Check sheet for the modelled part. Datum: model origin and axes. Units: mm. Coordinates: 2 decimals unless noted, no trailing zeros. Order: outer loops, then holes, each group sorted by start corner. A loop starts at its lowest first (then second) coordinate and runs counter-clockwise, first axis right, second up. Notation, with made-up numbers: (55, 48) -> (109, 48) arc R31 cw to (109, 82) -> close; hole circle Ø10 at (-6, 82). An arc over 180 degrees is marked (long way). Put each result on its own line as item: value. Start each with the question number.
```python
from build123d import *

# Parameters (mm, degrees)
F1_DEPTH = 6.35
F3_D     = 4.4958


with BuildPart() as f1:
    # F0 (on Front) → F1 (new body)
    with BuildSketch(Plane.XZ):
        with BuildLine():
            Line((18.2969275085, 15.24), (-18.2969275085, 15.24))
            ThreePointArc((-18.2969275085, 15.24), (0, -23.8125), (18.2969275085, 15.24))
        make_face()
    extrude(amount=F1_DEPTH)

    # F3 (through all)
    with Locations(Plane.XZ.offset(6.35)):
        with Locations((-15.7602855304, 9.525), (15.7602855304, 9.525), (-9.525, -15.7602855304), (9.525, -15.7602855304)):
            Hole(F3_D / 2)


solid = f1.part
```
1) Scan lines: line 1 along X through (y, z) = (-3.25, 8.5); line 2 along X through (y, z) = (-3.5, 9); line 3 along Z through (x, y) = (-17.5, -3). Record each from-to range of solid material in increasing order. Write a range as [from, to].
2) Sectioned sample at B-B (z = 8). Record the boundary of the cut face in (x, y).
3) Gauge pin test, flat ends, axial feed: pin 1 (1.5 mm diameter, centred on y = -2.5, z = 5, fed in from -X); pin 2 (3.5 mm diameter, centred on x = 15.76, z = 9.52, fed in from +Y); pin 3 (3 mm diameter, centred on y = -5.5, z = 7, fed in from +X); pin 4 (1 mm diameter, centred on y = -4, z = 1.5, fed in from +X). Record the tip position at first contact, or that the pin passes through.
4) Mould release check, pull along X, two halves, no side actions. Record for faces 1 (the cylindrical face through (-11.6, -3.13, -16.62)), 2 (the cylindrical face through (-0.8, -3.1, -23.8)), 3 (the flat face through (0, -3, 15.24)): +X half, -X half, draft (parallel to the pull), parting line (faces both ways), or undercut.
5) Sectioned sample at D-D (x = -9). Record the boundary of the cut face in (y, z).
6) Sectioned sample at A-A (x = -16). Record the boundary of the cut face in (y, z).
7) Sectioned sample at C-C (y = -1). Record the boundary of the cut face in (x, z) (1 decimal).
Entries:
1. line 1: x = [-22.24, -17.76], [-13.76, 13.76], [17.76, 22.24]
1. line 2: x = [-22.05, -17.95], [-13.57, 13.57], [17.95, 22.05]
1. line 3: z = [-16.15, 8.1], [10.95, 15.24]
2. outline: (-22.43, -6.35) -> (-17.41, -6.35) -> (-17.41, 0) -> (-22.43, 0) -> close; (-14.11, -6.35) -> (14.11, -6.35) -> (14.11, 0) -> (-14.11, 0) -> close; (17.41, -6.35) -> (22.43, -6.35) -> (22.43, 0) -> (17.41, 0) -> close
3. pin 1: stops at x = -23.43
3. pin 2: passes through
3. pin 3: stops at x = 23.17
3. pin 4: stops at x = 23.79
4. face 1: undercut
4. face 2: parting line
4. face 3: draft
5. outline: (-6.35, -22.05) -> (0, -22.05) -> (0, -17.95) -> (-6.35, -17.95) -> close; (-6.35, -13.57) -> (0, -13.57) -> (0, 15.24) -> (-6.35, 15.24) -> close
6. outline: (-6.35, -17.64) -> (0, -17.64) -> (0, 7.29) -> (-6.35, 7.29) -> close; (-6.35, 11.76) -> (0, 11.76) -> (0, 15.24) -> (-6.35, 15.24) -> close
7. outline: (-18.3, 15.2) arc R23.8 ccw (long way) to (18.3, 15.2) -> close; hole circle Ø4.5 at (-15.8, 9.5); hole circle Ø4.5 at (-9.5, -15.8); hole circle Ø4.5 at (9.5, -15.8); hole circle Ø4.5 at (15.8, 9.5)
